Input: dimensioned drawing with shaded views. Units: mm. Origin: part minimum x, y, z. A direction names the side the tool comes from. Coordinates: 2 decimals unless noted, no trailing zeros. Loops run counter-clockwise (first coordinate to the right, second up) from the corner with the lowest first, then second, coordinate; pieces in that order, holes last.
Item 1: Section A-A on z = 13.5. Return loops of the section in (x, y), and give its area (3 significant figures).
Item 2: Pull-direction query (X, two-part tool) for the marked faces 1, 2 and 3; classes: released by +X, released by -X, zero draft, split by the parting line, or undercut.
Item 3: Reachability of the marked faces 4 and 5 from +Z, -Z, +X, -X, +Y, -Y: full face, straight path, thin tool, end or side. Return the list, or none.
Item 4: Section B-B on x = 63.5. Return loops of the section in (y, z).
Item 5: Section D-D on x = 25.5. Return loops of the section in (y, z), and give its area (3 significant figures).
Item 6: Contact query for a flat-ended pin moving along its axis: P1, Ø1, axis at x = 26, y = 42, coming from the +Z side. Output: stop coordinate, or through.
Item 7: Section C-C on y = 21. Return loops of the section in (x, z), and give its area (3 significant figures).
Item 8: Ray query, line 1 along Y through (x, z) = (48, 14.5); line 2 along Z through (x, y) = (10, 42.5); line 3 along Y through (x, z) = (77, 14) (1 decimal). Return the intervals inside material, ascending.
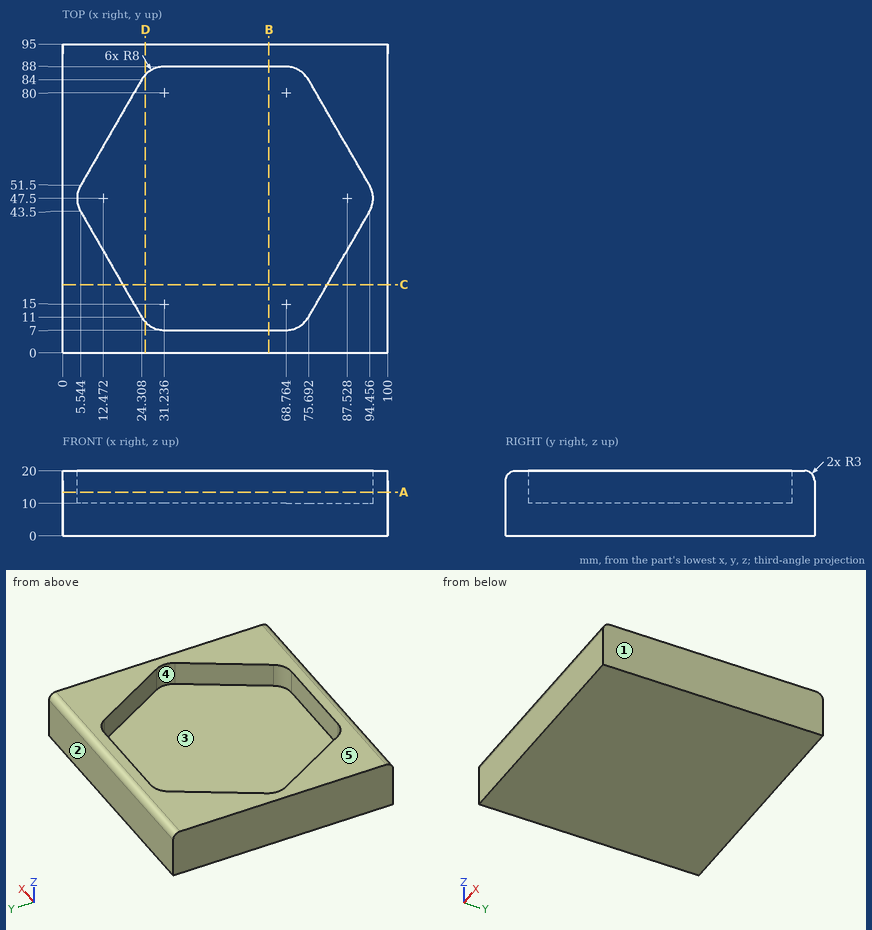
Results found:
1. outline: (0, 0) - (100, 0) - (100, 95) - (0, 95) - close; hole (5.54, 43.5) - (24.31, 11) arc R8 ccw to (31.24, 7) - (68.76, 7) arc R8 ccw to (75.69, 11) - (94.46, 43.5) arc R8 ccw to (94.46, 51.5) - (75.69, 84) arc R8 ccw to (68.76, 88) - (31.24, 88) arc R8 ccw to (24.31, 84) - (5.54, 51.5) arc R8 ccw to start
1. area: 3,840 mm2
2. face 1: released by +X
2. face 2: zero draft
2. face 3: undercut
3. face 4: +Z
3. face 5: +Z, +X, -X, +Y, -Y
4. outline: (0, 0) - (95, 0) - (95, 17) arc R3 ccw to (92, 20) - (88, 20) - (88, 10) - (7, 10) - (7, 20) - (3, 20) arc R3 ccw to (0, 17) - close
5. outline: (0, 0) - (95, 0) - (95, 17) arc R3 ccw to (92, 20) - (85.58, 20) - (85.58, 10) - (9.42, 10) - (9.42, 20) - (3, 20) arc R3 ccw to (0, 17) - close
5. area: 1,130 mm2
6. P1: stops at z = 10
7. outline: (0, 0) - (100, 0) - (100, 20) - (81.47, 20) - (81.47, 10) - (18.53, 10) - (18.53, 20) - (0, 20) - close
7. area: 1,370 mm2
8. line 1: y = 0 to 7, 88 to 95
8. line 2: z = 0 to 10
8. line 3: y = 0 to 13.3, 81.7 to 95
